The drawing under review shows one solid part. Ordinate dimensions are in mm from its lowest x, y, z. A direction names the side the tool comes from. Coordinates: 2 decimals unless noted, no trailing zeros. Order: outer loops, then holes, each group sorted by start corner. A loop starts at its lowest first (then second) coordinate and runs counter-clockwise, first axis right, second up. Notation, with made-up numbers: (89, -8.5) -> (143, -8.5) arc R22 ccw to (143, 4.5) -> close; hole circle Ø11 at (38, 65.25). An arc over 180 degrees is marked (long way). Use one line per item in the form item = value.
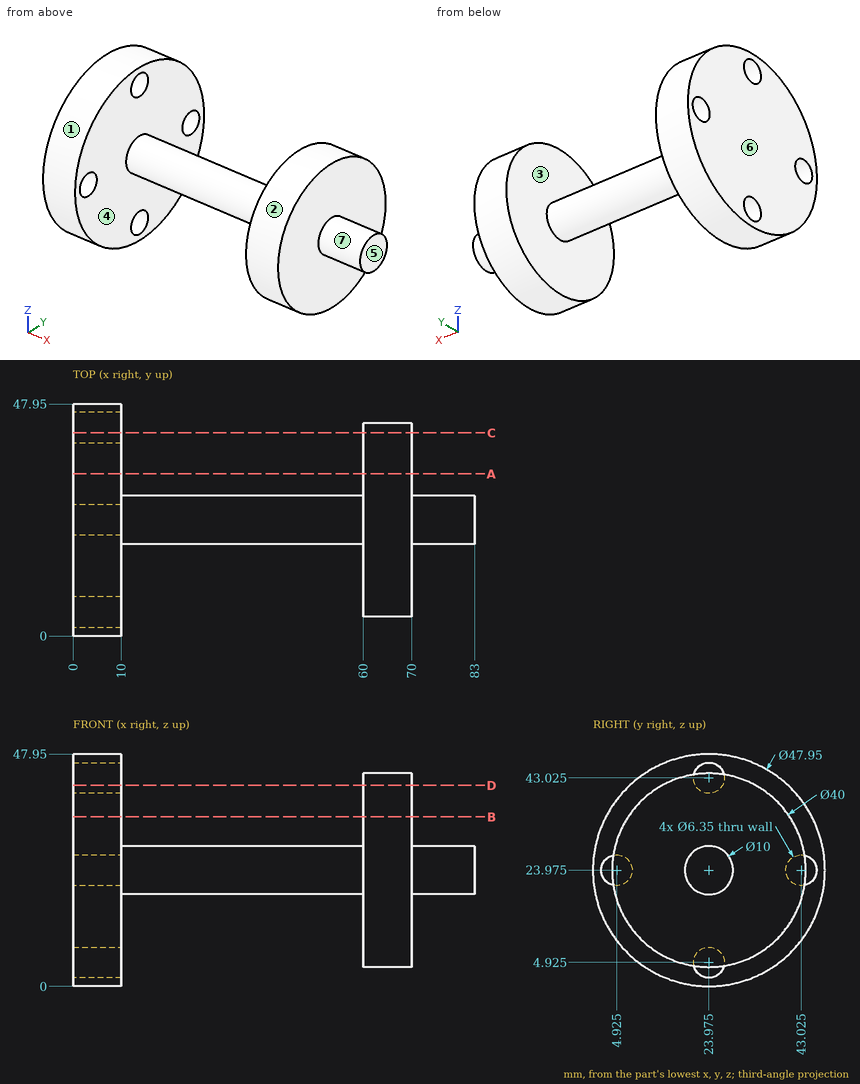
Item 1: We need section A-A (y = 33.5). Write out the cut boundary in (x, z), plus the area to 3 significant figures.
Results found:
outline = (0, 1.97) -> (10, 1.97) -> (10, 45.98) -> (0, 45.98) -> close; (60, 6.39) -> (70, 6.39) -> (70, 41.56) -> (60, 41.56) -> close
area = 792 mm²
Item 2: We need section B-B (z = 35). Write out the cut boundary in (x, y), plus the area to 3 significant figures.
Results found:
outline = (0, 2.69) -> (10, 2.69) -> (10, 45.26) -> (0, 45.26) -> close; (60, 7.29) -> (70, 7.29) -> (70, 40.66) -> (60, 40.66) -> close
area = 760 mm²
Item 3: Draft analysis for pull direction X (two halves, no side actions). For the marked faces 4, 5, 6 and 7, state which applies: released by +X, released by -X, zero draft, split by the parting line, or undercut.
Results found:
face_4 = undercut
face_5 = released by +X
face_6 = released by -X
face_7 = zero draft
Item 4: To check wall thickness, follow L1, parallel to X at y = 35, z = 9.5; L2, parallel to X at y = 34, z = 6.5; L3, parallel to Y at x = 6, z = 36.5. State the ranges of each line that lie inside material, in increasing order. Write a range as from..to.
Results found:
L1 = 0..10, 60..70
L2 = 0..10
L3 = 3.53..44.42
Item 5: Clearance check with flat-ended pins moving along their axes: pin 1 (4 mm diameter, centred on y = 23.975, z = 43.025, fed in from +X); pin 2 (5.5 mm diameter, centred on y = 43.025, z = 23.975, fed in from -X); pin 3 (4 mm diameter, centred on x = 59, y = 31.5, fed in from +Z); pin 4 (20 mm diameter, centred on y = 31, z = 24, fed in from +X). State where each tip first meets the part, or that it passes through.
Results found:
pin_1 = 70
pin_2 = 60
pin_3 = 43.12
pin_4 = 83
Item 6: We need section D-D (z = 41.5). Write out the cut boundary in (x, y).
Results found:
outline = (0, 7.61) -> (10, 7.61) -> (10, 21.19) -> (0, 21.19) -> close; (0, 26.76) -> (10, 26.76) -> (10, 40.34) -> (0, 40.34) -> close; (60, 14.34) -> (70, 14.34) -> (70, 33.61) -> (60, 33.61) -> close
Item 7: We need section C-C (y = 42). Write out the cut boundary in (x, z), plus the area to 3 significant figures.
Results found:
outline = (0, 8.17) -> (10, 8.17) -> (10, 20.97) -> (0, 20.97) -> close; (0, 26.98) -> (10, 26.98) -> (10, 39.78) -> (0, 39.78) -> close; (60, 15.31) -> (70, 15.31) -> (70, 32.64) -> (60, 32.64) -> close
area = 429 mm²
Item 8: Tool access review of the marked faces 1, 2 and 3: name each direction out of +Z, -Z, +X, -X, +Y, -Y from which nothing blocks a thin tool from reaching the whole face with its end or side.
Results found:
face_1 = +X, -X
face_2 = +X
face_3 = none
